Part model, mm, in its own coordinate system. A direction names the side the tool comes from. Round coordinates to 2 decimals unless told otherwise and drop trailing zeros. Write each loop counter-clockwise with the first axis right and the second up, starting at its lowest first coordinate (ties: lowest second). Pieces come first, ordered by that corner, then holes. Notation, with made-up numbers: M 69,4.5 L 105,4.5 A18 cw 105,12.5 Z; hole C 59,86 d4. An arc over 180 degrees is marked long. Answer as a JSON object with one key per item and string values. Group by question number.
1. Band-saw the part on D-D, the plane z = 2.5. Count the separate pieces of the cut face and the enclosed holes in it, plus the area to 3 significant figures.
2. Drop flat-ended pins along their axis: pin 1 (1.9 mm diameter, centred on x = -11, z = 2.5, fed in from -Y); pin 2 (1.9 mm diameter, centred on y = -9.5, z = 2.5, fed in from -X); pin 3 (2 mm diameter, centred on x = 4, z = 0.5, fed in from +Y). Give the stop position or say it passes through.
3. Band-saw the part on C-C, the plane y = -21. Write the cut outline in (x, z) (3 decimals).
4. Which spindle directions (+Z, -Z, +X, -X, +Y, -Y) get a long thin tool onto all of the face, cutting with end or side? Do faces 5 (the face through (-2.704, 2.684, 1.878)), 6 (the face through (-26.12, 1.83, 1.93)), 7 (the face through (3.639, 25.138, 1.878)). Say none if no direction does.
5. Two-plate mould, pull along Y, no slides. Class faces 1 (the face through (-21.001, -15.677, 1.932)), 2 (the face through (12.53, -23.02, 1.93)), 3 (the face through (0, 26.924, 2)), 4 (the face through (-16.62, 19.21, 1.88)): +Y half, -Y half, draft (parallel to the pull), parting line (faces both ways), or undercut.
6. Band-saw the part on B-B, the plane x = 4.5. Write the cut outline in (y, z) (3 decimals).
7. Drill centre lines: line 1 (Y direction, x = 15, z = 0.75) (3 decimals); line 2 (X direction, y = -13, z = 3.1) (3 decimals); line 3 (Y direction, x = 0, z = 1.6). Where is each one in solid material? Low to high. Write a range as from..to.
8. Band-saw the part on A-A, the plane y = 0. Write the cut outline in (x, z).
from build123d import *

# Parameters (mm, degrees)
SKETCH1_R           = 25.4
SKETCH1_R_2         = 0.9271
BOSS_EXTRUDE1_DEPTH = 3.81
BOSS_EXTRUDE2_DEPTH = 3.81


with BuildPart() as part:
    # Sketch1 → Boss-Extrude1 (new body)
    with BuildSketch(Plane.XY):
        Circle(SKETCH1_R)
        Circle(SKETCH1_R_2, mode=Mode.SUBTRACT)
        with BuildLine():
            Line((-1.905, 3.299556788), (-1.905, 22.143206633))
            ThreePointArc((-1.905, 22.143206633), (-15.715448212, 15.715448212), (-22.143206633, 1.905))
            Line((-22.143206633, 1.905), (-3.299556788, 1.905))
            ThreePointArc((-3.299556788, 1.905), (-2.694076836, 2.694076836), (-1.905, 3.299556788))
        make_face(mode=Mode.SUBTRACT)
        with BuildLine():
            Line((1.905, -22.143206633), (1.905, -3.299556788))
            ThreePointArc((1.905, -3.299556788), (2.694076836, -2.694076836), (3.299556788, -1.905))
            Line((3.299556788, -1.905), (22.143206633, -1.905))
            ThreePointArc((22.143206633, -1.905), (15.715448212, -15.715448212), (1.905, -22.143206633))
        make_face(mode=Mode.SUBTRACT)
        with BuildLine():
            Line((-1.905, -22.143206633), (-1.905, -3.299556788))
            ThreePointArc((-1.905, -3.299556788), (-2.694076836, -2.694076836), (-3.299556788, -1.905))
            Line((-3.299556788, -1.905), (-22.143206633, -1.905))
            ThreePointArc((-22.143206633, -1.905), (-15.715448212, -15.715448212), (-1.905, -22.143206633))
        make_face(mode=Mode.SUBTRACT)
        with BuildLine():
            Line((3.299556788, 1.905), (22.143206633, 1.905))
            ThreePointArc((22.143206633, 1.905), (15.715448212, 15.715448212), (1.905, 22.143206633))
            Line((1.905, 22.143206633), (1.905, 3.299556788))
            ThreePointArc((1.905, 3.299556788), (2.694076836, 2.694076836), (3.299556788, 1.905))
        make_face(mode=Mode.SUBTRACT)
    extrude(amount=BOSS_EXTRUDE1_DEPTH)

    # Sketch2 → Boss-Extrude2 (add)
    with BuildSketch(Plane.XY.offset(3.81)):
        with BuildLine():
            Line((5.308018177, 24.83918161), (5.757533246, 26.370089342))
            Line((5.757533246, 26.370089342), (9.413201475, 25.296688301))
            Line((9.413201475, 25.296688301), (8.963686407, 23.765780568))
            ThreePointArc((8.963686407, 23.765780568), (7.156006944, 24.37112153), (5.308018177, 24.83918161))
        make_face()
        with BuildLine():
            Line((-1.905, 25.328461757), (-1.905, 26.924))
            Line((-1.905, 26.924), (1.905, 26.924))
            Line((1.905, 26.924), (1.905, 25.328461757))
            ThreePointArc((1.905, 25.328461757), (0, 25.4), (-1.905, 25.328461757))
        make_face()
        with BuildLine():
            Line((12.091012289, 22.337578692), (12.953625389, 23.679830875))
            Line((12.953625389, 23.679830875), (16.158801349, 21.619989361))
            Line((16.158801349, 21.619989361), (15.296188249, 20.277737177))
            ThreePointArc((15.296188249, 20.277737177), (13.732276763, 21.367839734), (12.091012289, 22.337578692))
        make_face()
        with BuildLine():
            Line((17.894464494, 18.026317995), (19.100291842, 19.07117334))
            Line((19.100291842, 19.07117334), (21.595311238, 16.191767462))
            Line((21.595311238, 16.191767462), (20.38948389, 15.146912117))
            ThreePointArc((20.38948389, 15.146912117), (19.196039189, 16.633462642), (17.894464494, 18.026317995))
        make_face()
        with BuildLine():
            Line((22.248213608, 12.254672221), (23.699566243, 12.917482761))
            Line((23.699566243, 12.917482761), (25.282297443, 9.451784859))
            Line((25.282297443, 9.451784859), (23.830944807, 8.788974319))
            ThreePointArc((23.830944807, 8.788974319), (23.104652682, 10.55154133), (22.248213608, 12.254672221))
        make_face()
        with BuildLine():
            Line((24.79954477, 5.490225786), (26.378842734, 5.717294552))
            Line((26.378842734, 5.717294552), (26.921062268, 1.946074859))
            Line((26.921062268, 1.946074859), (25.341764304, 1.719006092))
            ThreePointArc((25.341764304, 1.719006092), (25.141464624, 3.614796892), (24.79954477, 5.490225786))
        make_face()
        with BuildLine():
            Line((25.341764304, -1.719006092), (26.921062268, -1.946074859))
            Line((26.921062268, -1.946074859), (26.378842734, -5.717294552))
            Line((26.378842734, -5.717294552), (24.79954477, -5.490225786))
            ThreePointArc((24.79954477, -5.490225786), (25.141464624, -3.614796892), (25.341764304, -1.719006092))
        make_face()
        with BuildLine():
            Line((23.830944807, -8.788974319), (25.282297443, -9.451784859))
            Line((25.282297443, -9.451784859), (23.699566243, -12.917482761))
            Line((23.699566243, -12.917482761), (22.248213608, -12.254672221))
            ThreePointArc((22.248213608, -12.254672221), (23.104652682, -10.55154133), (23.830944807, -8.788974319))
        make_face()
        with BuildLine():
            Line((20.38948389, -15.146912117), (21.595311238, -16.191767462))
            Line((21.595311238, -16.191767462), (19.100291842, -19.07117334))
            Line((19.100291842, -19.07117334), (17.894464494, -18.026317995))
            ThreePointArc((17.894464494, -18.026317995), (19.196039189, -16.633462642), (20.38948389, -15.146912117))
        make_face()
        with BuildLine():
            Line((15.296188249, -20.277737177), (16.158801349, -21.619989361))
            Line((16.158801349, -21.619989361), (12.953625389, -23.679830875))
            Line((12.953625389, -23.679830875), (12.091012289, -22.337578692))
            ThreePointArc((12.091012289, -22.337578692), (13.732276763, -21.367839734), (15.296188249, -20.277737177))
        make_face()
        with BuildLine():
            Line((8.963686407, -23.765780568), (9.413201475, -25.296688301))
            Line((9.413201475, -25.296688301), (5.757533246, -26.370089342))
            Line((5.757533246, -26.370089342), (5.308018177, -24.83918161))
            ThreePointArc((5.308018177, -24.83918161), (7.156006944, -24.37112153), (8.963686407, -23.765780568))
        make_face()
        with BuildLine():
            Line((1.905, -25.328461757), (1.905, -26.924))
            Line((1.905, -26.924), (-1.905, -26.924))
            Line((-1.905, -26.924), (-1.905, -25.328461757))
            ThreePointArc((-1.905, -25.328461757), (0, -25.4), (1.905, -25.328461757))
        make_face()
        with BuildLine():
            Line((-5.308018177, -24.83918161), (-5.757533246, -26.370089342))
            Line((-5.757533246, -26.370089342), (-9.413201475, -25.296688301))
            Line((-9.413201475, -25.296688301), (-8.963686407, -23.765780568))
            ThreePointArc((-8.963686407, -23.765780568), (-7.156006944, -24.37112153), (-5.308018177, -24.83918161))
        make_face()
        with BuildLine():
            Line((-12.091012289, -22.337578692), (-12.953625389, -23.679830875))
            Line((-12.953625389, -23.679830875), (-16.158801349, -21.619989361))
            Line((-16.158801349, -21.619989361), (-15.296188249, -20.277737177))
            ThreePointArc((-15.296188249, -20.277737177), (-13.732276763, -21.367839734), (-12.091012289, -22.337578692))
        make_face()
        with BuildLine():
            Line((-17.894464494, -18.026317995), (-19.100291842, -19.07117334))
            Line((-19.100291842, -19.07117334), (-21.595311238, -16.191767462))
            Line((-21.595311238, -16.191767462), (-20.38948389, -15.146912117))
            ThreePointArc((-20.38948389, -15.146912117), (-19.196039189, -16.633462642), (-17.894464494, -18.026317995))
        make_face()
        with BuildLine():
            Line((-22.248213608, -12.254672221), (-23.699566243, -12.917482761))
            Line((-23.699566243, -12.917482761), (-25.282297443, -9.451784859))
            Line((-25.282297443, -9.451784859), (-23.830944807, -8.788974319))
            ThreePointArc((-23.830944807, -8.788974319), (-23.104652682, -10.55154133), (-22.248213608, -12.254672221))
        make_face()
        with BuildLine():
            Line((-24.79954477, -5.490225786), (-26.378842734, -5.717294552))
            Line((-26.378842734, -5.717294552), (-26.921062268, -1.946074859))
            Line((-26.921062268, -1.946074859), (-25.341764304, -1.719006092))
            ThreePointArc((-25.341764304, -1.719006092), (-25.141464624, -3.614796892), (-24.79954477, -5.490225786))
        make_face()
        with BuildLine():
            Line((-25.341764304, 1.719006092), (-26.921062268, 1.946074859))
            Line((-26.921062268, 1.946074859), (-26.378842734, 5.717294552))
            Line((-26.378842734, 5.717294552), (-24.79954477, 5.490225786))
            ThreePointArc((-24.79954477, 5.490225786), (-25.141464624, 3.614796892), (-25.341764304, 1.719006092))
        make_face()
        with BuildLine():
            Line((-23.830944807, 8.788974319), (-25.282297443, 9.451784859))
            Line((-25.282297443, 9.451784859), (-23.699566243, 12.917482761))
            Line((-23.699566243, 12.917482761), (-22.248213608, 12.254672221))
            ThreePointArc((-22.248213608, 12.254672221), (-23.104652682, 10.55154133), (-23.830944807, 8.788974319))
        make_face()
        with BuildLine():
            Line((-20.38948389, 15.146912117), (-21.595311238, 16.191767462))
            Line((-21.595311238, 16.191767462), (-19.100291842, 19.07117334))
            Line((-19.100291842, 19.07117334), (-17.894464494, 18.026317995))
            ThreePointArc((-17.894464494, 18.026317995), (-19.196039189, 16.633462642), (-20.38948389, 15.146912117))
        make_face()
        with BuildLine():
            Line((-15.296188249, 20.277737177), (-16.158801349, 21.619989361))
            Line((-16.158801349, 21.619989361), (-12.953625389, 23.679830875))
            Line((-12.953625389, 23.679830875), (-12.091012289, 22.337578692))
            ThreePointArc((-12.091012289, 22.337578692), (-13.732276763, 21.367839734), (-15.296188249, 20.277737177))
        make_face()
        with BuildLine():
            Line((-8.963686407, 23.765780568), (-9.413201475, 25.296688301))
            Line((-9.413201475, 25.296688301), (-5.757533246, 26.370089342))
            Line((-5.757533246, 26.370089342), (-5.308018177, 24.83918161))
            ThreePointArc((-5.308018177, 24.83918161), (-7.156006944, 24.37112153), (-8.963686407, 23.765780568))
        make_face()
    extrude(amount=-BOSS_EXTRUDE2_DEPTH)


solid = part.part
Worked answers:
{
 "1": {"separate pieces": "1", "enclosed holes": "5", "area": "930 mm^2"},
 "2": {"pin 1": "stops at y = -23.33", "pin 2": "stops at x = -25.28", "pin 3": "stops at y = 25.22"},
 "3": {"outline": "M -15.76,0 L -7.277,0 L -7.277,3.81 L -15.76,3.81 Z; M -1.905,0 L 1.905,0 L 1.905,3.81 L -1.905,3.81 Z; M 7.277,0 L 15.76,0 L 15.76,3.81 L 7.277,3.81 Z"},
 "4": {"face 5": "+Z, -Z", "face 6": "+Z, -Z, -X", "face 7": "+Z, -Z, +Y"},
 "5": {"face 1": "undercut", "face 2": "-Y half", "face 3": "+Y half", "face 4": "undercut"},
 "6": {"outline": "M -24.998,0 L -21.765,0 L -21.765,3.81 L -24.998,3.81 Z; M -1.905,0 L 1.905,0 L 1.905,3.81 L -1.905,3.81 Z; M 21.765,0 L 24.998,0 L 24.998,3.81 L 21.765,3.81 Z"},
 "7": {"line 1": "y = -22.365..-16.4, -1.905..1.905, 16.4..22.365", "line 2": "x = -21.821..-18.026, -1.905..1.905, 18.026..21.821", "line 3": "y = -26.92..-0.93, 0.93..26.92"},
 "8": {"outline": "M -25.4,0 L -0.93,0 L -0.93,3.81 L -25.4,3.81 Z; M 0.93,0 L 25.4,0 L 25.4,3.81 L 0.93,3.81 Z"}
}
